Here's how the part is built. I have some questions about the finished solid (model axes, mm). A direction names the side the tool comes from. Coordinates: 2 decimals unless noted, no trailing zeros. Write each loop counter-clockwise with the first axis right and the second up, starting at its lowest first coordinate (ties: lowest second). Pieces come first, ordered by that corner, then holes. Notation, with made-up numbers: (33, 64.5) -> (44, 64.5) arc R23 cw to (44, 77.5) -> close; hole circle Ø11 at (54.5, 18). An arc over 180 degrees is marked (long way). Use a Markdown table: item, result. Add a question column.
Item 1: Imagine slicing it at D-D, the plane y = 6. Write out the boundary of the cut face in (x, z), and give its area (3 significant figures).
Item 2: Imagine slicing it at A-A, the plane x = -0.25. Write out the boundary of the cut face in (y, z).
Item 3: If I drill on line 1 along Y through (x, z) = (5.25, 132); line 2 along Y through (x, z) = (-13.5, 85.5); line 3 along Z through (x, y) = (-2.75, 2.5), over which ranges is the centre line in solid material (lowest first)? Write a range as from..to.
Item 4: On a 3-axis mill with a long thin cutter (end or side, diameter ignored), from which of +Z, -Z, +X, -X, +Y, -Y can I reach the whole of each face in a straight line? I mean faces 5 (the cylindrical face through (0, 0, 15)), 6 (the flat face through (0, 0, 157)). Say none if no direction works.
Item 5: Will this pin go through, and if not, where does the flat tip stop? pin 1 Ø17.5 at (y, z) = (0, 132) entering from +X.
Item 6: Imagine slicing it at B-B, the plane y = 0. Write out the boundary of the cut face in (x, z).
Item 7: If we mould it in two halves opening along Y, with no side actions, what happens to faces 1 (the cylindrical face through (0, 0, 143)), 2 (the cylindrical face through (0, 0, 102)), 3 (the flat face through (0, -25, 77)), 4 (the flat face through (0, 0, 0))? For each: pulls with the +Y half, pulls with the -Y half, needs draft (parallel to the pull), parting line crosses it, or undercut.
Item 8: Imagine slicing it at C-C, the plane z = 65. Write out the boundary of the cut face in (x, y).
Autodesk Inventor part; units mm, degrees
ref_plane "Startebene" through (0, 0, 0) normal (0, 0, 1) x (1, 0, 0)
ref_plane "Endebene" through (0, 0, 157) normal (0, 0, 1) x (1, 0, 0)
ref_plane "YZ Plane" through (0, 0, 0) normal (1, 0, 0) x (0, 1, 0)
ref_plane "Startebene" through (0, 0, 0) normal (0, 0, 1) x (1, 0, 0)
ref_plane "Endebene" through (0, 0, 157) normal (0, 0, 1) x (1, 0, 0)
sketch "Skizze" plane through (0, 0, 0) normal (0, 0, 1) x (1, 0, 0)
  line L0 (15, -25) -> (-15, -25)
  line L1 (-15, -25) -> (-15, 25)
  line L2 (-15, 25) -> (15, 25)
  line L3 (15, 25) -> (15, -25)
  line L4 (-6, 0) -> (8, 0) construction
  line L5 (0, -30) -> (0, 40) construction
  line L6 (0, 54) -> (0, -44) construction
  line L7 (-9.2, 0) -> (13.2, 0) construction
  dimension "d0" = 50
  dimension "d1" = 30
  dimension "d4" = 15
  dimension "d5" = 25
extrude "Körper" add sketch "Skizze" along normal up to surface (157 mm away) from surface at 0
sketch "Sketch3" plane through (0, 0, 0) normal (0, 0, 1) x (1, 0, 0)
  line L0 (0, 0) -> (10, 0)
ref_plane "Work Plane3" through (0, 0, 0) normal (0, -1, 0) x (1, 0, 0)
sketch "Sketch4" plane through (0, 0, 0) normal (0, -1, 0) x (1, 0, 0)
  line L0 (-2, 0) -> (12, 0)
  line L1 (-2, 157) -> (12, 157)
  dimension "d9" = 157
sketch "Skizze5" plane through (15, -25, 157) normal (1, 0, 0) x (0, 0, -1)
  line L0 (157, 50) -> (0, 50)
  circle A0 centre (25, 25) radius 11
  arc A1 (70, 40) -> (70, 10) centre (70, 25) ccw
  arc A2 (127, 10) -> (127, 40) centre (127, 25) ccw
  line L1 (70, 40) -> (127, 40)
  line L2 (70, 10) -> (127, 10)
  line L3 (0, 50) -> (0, 0)
  point P0 (157, 25)
  dimension "d10" = 57
  dimension "d11" = 30
  dimension "d14" = 22
  dimension "d15" = 25
  dimension "d16" = 25
  dimension "d19" = 70
  dimension "d21" = 25
extrude "Extrusion2" cut sketch "Skizze5" against normal up to next
equation "\"d0\" = G_W"
equation "\"d1\" = G_H"
equation "\"d4\" = 0.5 * d1"
equation "\"d5\" = 0.5 * d0"
equation "\"d2\" = G_L"
equation "\"G_W\" = 50"
equation "\"G_H\" = 30"
equation "\"G_L\" = d9"
equation "\"G_OFFSET_START\" = 0"
equation "\"G_OFFSET_END\" = 0"
equation "\"d7\" = G_OFFSET_END + B_L"
equation "\"B_L\" = 157"
properties part number "EN 10058 - 50 x 30 - 157" material "Stahl, weich"
Ans:
| question | item | result |
|---|---|---|
| 1 | outline | (-15, 0) -> (15, 0) -> (15, 16.25) -> (-15, 16.25) -> close; (-15, 100.75) -> (15, 100.75) -> (15, 122.78) -> (-15, 122.78) -> close; (-15, 141.22) -> (15, 141.22) -> (15, 157) -> (-15, 157) -> close |
| 1 | area | 1,620 mm^2 |
| 2 | outline | (-25, 0) -> (25, 0) -> (25, 157) -> (-25, 157) -> close; hole (-15, 30) arc R15 ccw to (15, 30) -> (15, 87) arc R15 ccw to (-15, 87) -> close; hole circle Ø22 at (0, 132) |
| 3 | line 1 | y = -25..-11, 11..25 |
| 3 | line 2 | y = -25..-15, 15..25 |
| 3 | line 3 | z = 0..15.21, 101.79..121.29, 142.71..157 |
| 4 | face 5 | +X, -X |
| 4 | face 6 | +Z, +X, -X, +Y, -Y |
| 5 | pin 1 | passes through |
| 6 | outline | (-15, 0) -> (15, 0) -> (15, 15) -> (-15, 15) -> close; (-15, 102) -> (15, 102) -> (15, 121) -> (-15, 121) -> close; (-15, 143) -> (15, 143) -> (15, 157) -> (-15, 157) -> close |
| 7 | face 1 | undercut |
| 7 | face 2 | undercut |
| 7 | face 3 | pulls with the -Y half |
| 7 | face 4 | needs draft |
| 8 | outline | (-15, -25) -> (15, -25) -> (15, -15) -> (-15, -15) -> close; (-15, 15) -> (15, 15) -> (15, 25) -> (-15, 25) -> close |
